Verification items for the finished model (mm, model axes). A direction names the side the tool comes from. Give positions to 0.01 mm unless a question says otherwise; leave off trailing zeros. Loops run counter-clockwise (first coordinate to the right, second up) from the corner with the lowest first, then second, coordinate; pieces in that order, holes last. Notation, with made-up numbers: M -2,-29 L 52,-29 A22 cw 52,-23 Z; hole C 11,88.5 d9. An arc over 180 degrees is marked long. Use CSV: the item, a comma, the result in double quotes.
from build123d import *

# Parameters (mm, degrees)
F0_W     = 10
F0_H     = 10
F1_DEPTH = 5
F2_R     = 4.99999


# Not quite as in the source:
# - a fillet or chamfer is up to 0.001 mm smaller than in the source, because OpenCascade refuses the exact size
# - a feature names something its author has since deleted; it is built from what else it names


with BuildPart() as f1:
    # F0 (on Top) → F1 (new body)
    with BuildSketch(Plane.XY):
        Polygon((15, 65), (-15, 65), (-15, 55), (-5, 55), (5, 55), (15, 55), align=None)
        with Locations((0, 50)):
            Rectangle(F0_W, F0_H)
        Polygon((5, 45), (-5, 45), (-18.6396103068, 45), (18.6396103068, -45), (28.2842712475, -35.3553390593), (35.3553390593, -28.2842712475), (45, -18.6396103068), (45, -5), (45, 5), (45, 18.6396103068), (35.3553390593, 28.2842712475), (28.2842712475, 35.3553390593), (18.6396103068, 45), align=None)
        Polygon((18.6396103068, -45), (-18.6396103068, 45), (-28.2842712475, 35.3553390593), (-35.3553390593, 28.2842712475), (-45, 18.6396103068), (-45, 5), (-45, -5), (-45, -18.6396103068), (-35.3553390593, -28.2842712475), (-28.2842712475, -35.3553390593), (-18.6396103068, -45), (-5, -45), (5, -45), align=None)
        Polygon((-35.3553390593, 28.2842712475), (-28.2842712475, 35.3553390593), (-35.3553390593, 42.4264068712), (-42.4264068712, 35.3553390593), align=None)
        Polygon((35.3553390593, 42.4264068712), (28.2842712475, 35.3553390593), (35.3553390593, 28.2842712475), (42.4264068712, 35.3553390593), align=None)
        Polygon((-42.4264068712, 35.3553390593), (-35.3553390593, 42.4264068712), (-28.2842712475, 49.4974746831), (-35.3553390593, 56.5685424949), (-56.5685424949, 35.3553390593), (-49.4974746831, 28.2842712475), align=None)
        with Locations((0, -50)):
            Rectangle(F0_W, F0_H)
        Polygon((35.3553390593, -28.2842712475), (28.2842712475, -35.3553390593), (35.3553390593, -42.4264068712), (42.4264068712, -35.3553390593), align=None)
        Polygon((28.2842712475, 49.4974746831), (35.3553390593, 42.4264068712), (42.4264068712, 35.3553390593), (49.4974746831, 28.2842712475), (56.5685424949, 35.3553390593), (35.3553390593, 56.5685424949), align=None)
        Polygon((15, -55), (5, -55), (-5, -55), (-15, -55), (-15, -65), (15, -65), align=None)
        Polygon((42.4264068712, -35.3553390593), (35.3553390593, -42.4264068712), (28.2842712475, -49.4974746831), (35.3553390593, -56.5685424949), (56.5685424949, -35.3553390593), (49.4974746831, -28.2842712475), align=None)
        with Locations((-50, 0)):
            Rectangle(F0_W, F0_H)
        with Locations((50, 0)):
            Rectangle(F0_W, F0_H)
        Polygon((-55, -5), (-55, 5), (-55, 15), (-65, 15), (-65, -15), (-55, -15), align=None)
        Polygon((-35.3553390593, -42.4264068712), (-28.2842712475, -35.3553390593), (-35.3553390593, -28.2842712475), (-42.4264068712, -35.3553390593), align=None)
        Polygon((55, 15), (55, 5), (55, -5), (55, -15), (65, -15), (65, 15), align=None)
        Polygon((-28.2842712475, -49.4974746831), (-35.3553390593, -42.4264068712), (-42.4264068712, -35.3553390593), (-49.4974746831, -28.2842712475), (-56.5685424949, -35.3553390593), (-35.3553390593, -56.5685424949), align=None)
    extrude(amount=F1_DEPTH)

    # F2 (radius 5 in the source; OpenCascade refuses exactly that, so slightly less here)
    f2_edges = [f1.edges().sort_by_distance(p)[0] for p in [
        (65, 15, 2.5),
        (65, -15, 2.5),
        (55, 15, 2.5),
        (55, -15, 2.5),
    ]]
    fillet(f2_edges, radius=F2_R)


solid = f1.part
(1) Section check A-A on y = 37. Record the cut outline in (x, z), plus the area to 3 significant figures.
Calculated:
outline,"M -54.92,0 L -29.93,0 L -29.93,5 L -54.92,5 Z; M -26.64,0 L 26.64,0 L 26.64,5 L -26.64,5 Z; M 29.93,0 L 54.92,0 L 54.92,5 L 29.93,5 Z"
area,"516 mm²"
(2) Tool access check on faces 1 (the flat face through (-31.869, -53.083, 2.465)), 2 (the flat face through (46.11, 45.813, 2.465)), 3 (the flat face through (38.84, 31.77, 2.46)), 4 (the flat face through (40.11, -23.53, 2.46)), 5 (the cylindrical face through (63, -14, 3)). Record the directions out of +Z, -Z, +X, -X, +Y, -Y that give a thin tool (end or side, any length) a straight path to the whole face; none if there is none.
Calculated:
face 1,"+Z, -Z, -Y"
face 2,"+Z, -Z, +X, +Y"
face 3,"+Z, -Z"
face 4,"+Z, -Z, +X"
face 5,"+Z, -Z, +X, -Y"
(3) Scan lines: L1, parallel to Y at x = 7, z = 2.15; L2, parallel to X at y = -35, z = 1.05. Record each from-to range of solid material in increasing order. Write a range as from..to.
Calculated:
L1,"y = -65..-55, -45..45, 55..65"
L2,"x = -56.21..-42.78, -42.07..42.07, 42.78..56.21"
(4) Depth check by flat-ended pin: pin 1 Ø1.5 at (y, z) = (62, 2.5) entering from +X; pin 2 Ø3 at (y, z) = (-44.5, 3.5) entering from -X; pin 3 Ø2.5 at (y, z) = (49, 2) entering from +X; pin 4 Ø8 at (x, y) = (-20, -47) entering from -Z. Enter the tip coordinate at first touch or a pass-through.
Calculated:
pin 1,"stops at x = 15"
pin 2,"stops at x = -48.92"
pin 3,"stops at x = 44.17"
pin 4,"stops at z = 0"
(5) Section check B-B on x = -10.5. Record the cut outline in (y, z).
Calculated:
outline,"M -65,0 L -55,0 L -55,5 L -65,5 Z; M -45,0 L 45,0 L 45,5 L -45,5 Z; M 55,0 L 65,0 L 65,5 L 55,5 Z"
(6) Mould release check, pull along Y, two halves, no side actions. Record for faces 6 (the cylindrical face through (64, 13, 3)), 7 (the flat face through (-52.984, -31.77, 2.465)), 8 (the flat face through (65, 0, 2)): released by +Y, released by -Y, zero draft, split by the parting line, or undercut.
Calculated:
face 6,"released by +Y"
face 7,"undercut"
face 8,"zero draft"
